from build123d import *

# Parameters (mm, degrees)
F0_R     = 1.443985
F0_R_2   = 0.5
F1_DEPTH = 1
F2_DEPTH = 12.5
F3_DEPTH = 1


with BuildPart() as f1:
    # F0 (on Top) → F1 (new body, symmetric)
    with BuildSketch(Plane.XY):
        with BuildLine():
            Line((-30.798228, 29.969801), (-15.828427, 15))
            Line((-15.828427, 15), (-13, 15))
            Line((-13, 15), (-31.713203, 33.713203))
            ThreePointArc((-31.713203, 33.713203), (-32.093806, 31.799786), (-33.17767, 30.17767))
            ThreePointArc((-33.17767, 30.17767), (-34.799786, 29.093806), (-36.713203, 28.713203))
            Line((-36.713203, 28.713203), (-18, 10))
            Line((-18, 10), (-18, 12.828427))
            Line((-18, 12.828427), (-32.969801, 27.798228))
            add(Edge.make_bspline(
                [(-32.969801, 27.798228), (-32.001644, 27.823906), (-30.61594, 29.101571), (-30.798228, 29.969801)],
                knots=[0, 0, 0, 0, 3.071068, 3.071068, 3.071068, 3.071068], degree=3))
        make_face()
        Polygon((0, 15), (-13, 15), (-18, 10), (-18, 0), (0, 0), align=None)
        with Locations((-10, 10)):
            Circle(F0_R, mode=Mode.SUBTRACT)
        Polygon((-15.828427, 15), (-18, 15), (-18, 12.828427), (-18, 10), (-13, 15), align=None)
        with BuildLine():
            ThreePointArc((-33.17767, 30.17767), (-32.093806, 31.799786), (-31.713203, 33.713203))
            Line((-31.713203, 33.713203), (-34.213203, 36.213203))
            Line((-34.213203, 36.213203), (-36.713203, 33.713203))
            Line((-36.713203, 33.713203), (-33.17767, 30.17767))
        make_face()
        with Locations((-33.884776, 33.713203)):
            Circle(F0_R_2, mode=Mode.SUBTRACT)
        with BuildLine():
            Line((-34.213203, 36.213203), (-31.713203, 33.713203))
            ThreePointArc((-31.713203, 33.713203), (-34.799786, 38.332601), (-40.248737, 37.248737))
            Line((-40.248737, 37.248737), (-36.713203, 33.713203))
            Line((-36.713203, 33.713203), (-34.213203, 36.213203))
        make_face()
        with Locations((-36.713203, 36.541631)):
            Circle(F0_R_2, mode=Mode.SUBTRACT)
        with BuildLine():
            Line((-18, 12.828427), (-18, 15))
            Line((-18, 15), (-15.828427, 15))
            Line((-15.828427, 15), (-30.798228, 29.969801))
            add(Edge.make_bspline(
                [(-32.969801, 27.798228), (-32.001644, 27.823906), (-30.61594, 29.101571), (-30.798228, 29.969801)],
                knots=[0, 0, 0, 0, 3.071068, 3.071068, 3.071068, 3.071068], degree=3))
            Line((-32.969801, 27.798228), (-18, 12.828427))
        make_face()
        with BuildLine():
            Line((-39.213203, 31.213203), (-36.713203, 28.713203))
            ThreePointArc((-36.713203, 28.713203), (-34.799786, 29.093806), (-33.17767, 30.17767))
            Line((-33.17767, 30.17767), (-36.713203, 33.713203))
            Line((-36.713203, 33.713203), (-39.213203, 31.213203))
        make_face()
        with Locations((-36.713203, 30.884776)):
            Circle(F0_R_2, mode=Mode.SUBTRACT)
        with BuildLine():
            ThreePointArc((-40.248737, 37.248737), (-41.332601, 31.799786), (-36.713203, 28.713203))
            Line((-36.713203, 28.713203), (-39.213203, 31.213203))
            Line((-39.213203, 31.213203), (-36.713203, 33.713203))
            Line((-36.713203, 33.713203), (-40.248737, 37.248737))
        make_face()
        with Locations((-39.541631, 33.713203)):
            Circle(F0_R_2, mode=Mode.SUBTRACT)
        with Locations((-36.713203, 30.884776)):
            Circle(F0_R_2)
        with Locations((-33.884776, 33.713203)):
            Circle(F0_R_2)
        with Locations((-39.541631, 33.713203)):
            Circle(F0_R_2)
        with Locations((-36.713203, 36.541631)):
            Circle(F0_R_2)
    extrude(amount=F1_DEPTH, both=True)

    # F0 (on Top) → F2 (cut, symmetric)
    with BuildSketch(Plane.XY):
        with Locations((-39.541631, 33.713203)):
            Circle(F0_R_2)
        with Locations((-36.713203, 36.541631)):
            Circle(F0_R_2)
        with Locations((-33.884776, 33.713203)):
            Circle(F0_R_2)
        with Locations((-36.713203, 30.884776)):
            Circle(F0_R_2)
    extrude(amount=F2_DEPTH, both=True, mode=Mode.SUBTRACT)

    # F0 (on Top) → F3 (cut)
    with BuildSketch(Plane.XY):
        with BuildLine():
            Line((-18, 12.828427), (-18, 15))
            Line((-18, 15), (-15.828427, 15))
            Line((-15.828427, 15), (-30.798228, 29.969801))
            add(Edge.make_bspline(
                [(-32.969801, 27.798228), (-32.001644, 27.823906), (-30.61594, 29.101571), (-30.798228, 29.969801)],
                knots=[0, 0, 0, 0, 3.071068, 3.071068, 3.071068, 3.071068], degree=3))
            Line((-32.969801, 27.798228), (-18, 12.828427))
        make_face()
    extrude(amount=F3_DEPTH, mode=Mode.SUBTRACT)

    # F4: F1 across plane


with BuildPart() as f1_1:
    add(f1.part)
    add(f1.part.mirror(Plane.XZ))

    # F5: F1 across plane


with BuildPart() as f1_2:
    add(f1_1.part)
    add(f1_1.part.mirror(Plane.YZ))


solid = f1_2.part
The listing builds one solid part. Answer for the finished solid, in the listing's coordinates (mm). A direction names the side the tool comes from. Round coordinates to 2 decimals unless told otherwise and drop trailing zeros. Write each loop counter-clockwise with the first axis right and the second up, starting at its lowest first coordinate (ties: lowest second). Pieces come first, ordered by that corner, then holes. Notation, with made-up numbers: M -30,68 L 13,68 A9 cw 13,73 Z; hole C 89.25,47.25 d5. An arc over 180 degrees is marked long. Write each question's results on one line, items separated by ' | '. Start each with the question number.
(1) The part is cut by section A-A, the plane x = 10. Write down the section's boundary in (y, z), and give its area (3 significant figures).
(2) The part is cut by section B-B, the plane y = 23.5. Write down the section's boundary in (x, z), and give its area (3 significant figures).
(3) Find the intervals of material crossed by line 1 (Y direction, x = 10, z = 0.5); line 2 (X direction, y = -10, z = 0.35); line 3 (X direction, y = -15.5, z = 0.7), in increasing order.
(4) For faces 5 (the flat face through (18, 0, 0)), 6 (the flat face through (23.21, 22.38, 0.49)), 7 (the flat face through (-18, 0, 0)), 8 (the flat face through (-22, -24, 0)), determine the directions among +Z, -Z, +X, -X, +Y, -Y from which every point of the face is accessible in a straight line to the end or side of a thin tool.
(5) Determine the mould class of faces 1 (the flat face through (27, 19, 0)), 2 (the flat face through (22, -24, 0)), 3 (the flat face through (-23.21, -22.38, 0.49)), 4 (the flat face through (-27, -19, 0)) for opening direction X: +X half, -X half, draft (parallel to the pull), parting line (faces both ways), or undercut.
(6) Each of these flat-tipped pins is pushed along its axis until it touches: P1, Ø2.5, axis at x = -10, y = -10, coming from the -Z side; P2, Ø0.5, axis at y = -14.5, z = 0.5, coming from the -X side; P3, Ø1.1, axis at x = 17.5, z = 0.5, coming from the +Y side; P4, Ø0.6, axis at x = -2, z = 0.5, coming from the +Y side. Where does it stop, or does it pass through?
(7) The part is cut by section C-C, the plane x = 27. Write down the section's boundary in (y, z).
(8) The part is cut by section D-D, the plane y = 4. Write down the section's boundary in (x, z), and give its area (3 significant figures).
Worked answers:
1) outline: M -15,-1 L -11.44,-1 L -11.44,1 L -15,1 Z; M -8.56,-1 L 8.56,-1 L 8.56,1 L -8.56,1 Z; M 11.44,-1 L 15,-1 L 15,1 L 11.44,1 Z | area: 48.4 mm²
2) outline: M -31.5,-1 L -21.5,-1 L -21.5,1 L -24.33,1 L -24.33,0 L -28.67,0 L -28.67,1 L -31.5,1 Z; M 21.5,-1 L 31.5,-1 L 31.5,1 L 28.67,1 L 28.67,0 L 24.33,0 L 24.33,1 L 21.5,1 Z | area: 31.3 mm²
3) line 1: y = -15 to -11.44, -8.56 to 8.56, 11.44 to 15 | line 2: x = -18 to -11.44, -8.56 to 8.56, 11.44 to 18 | line 3: x = -23.5 to -20.67, -16.33 to -13.5, 13.5 to 16.33, 20.67 to 23.5
4) face 5: +Z, -Z, +X | face 6: +Z | face 7: +Z, -Z, -X | face 8: +Z, -Z, -Y
5) face 1: +X half | face 2: undercut | face 3: undercut | face 4: -X half
6) P1: passes through | P2: stops at x = -22.75 | P3: stops at y = 20.05 | P4: stops at y = 15
7) outline: M -29,-1 L -19,-1 L -19,1 L -21.83,1 L -21.83,0 L -26.17,0 L -26.17,1 L -29,1 Z; M 19,-1 L 29,-1 L 29,1 L 26.17,1 L 26.17,0 L 21.83,0 L 21.83,1 L 19,1 Z
8) outline: M -18,-1 L 18,-1 L 18,1 L -18,1 Z | area: 72.0 mm²
